Check sheet for the drawn part. Datum: minimum x, y, z corner. Units: mm. Give positions to 0.01 mm unless a question says otherwise; leave off trailing zeros. Loops run counter-clockwise (first coordinate to the right, second up) from the corner with the lowest first, then second, coordinate; pieces in that order, holes last.
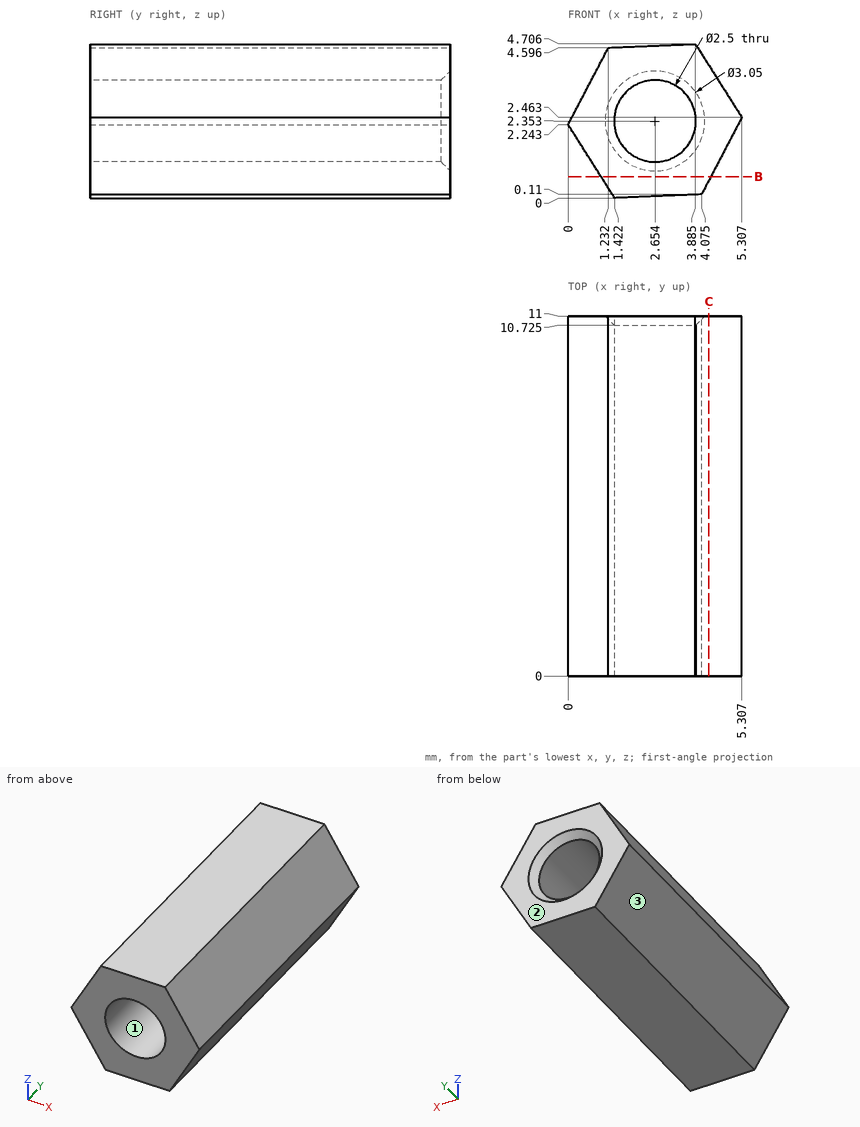
(1) Release check for a two-part mould opening along Z. For the marked faces 1, 2 and 3 record: pulls with the +Z half, pulls with the -Z half, needs draft (parallel to the pull), parting line crosses it, or undercut.
(2) Section check C-C on x = 4.3. Record the boundary of the cut face in (y, z).
(3) Material ranges on line 1 (Z direction, x = 1.7, y = 10) (1 decimal); line 2 (Z direction, x = 2.6, y = 9.25) (1 decimal); line 3 (X direction, y = 1.25, z = 3.35) (1 decimal), recorded low to high.
(4) Gauge pin test, flat end, axial feed: pin 1 Ø1 at (y, z) = (7, 1.5) entering from +X (1 decimal). Record the tip position at first contact, or that the pin passes through.
(5) Section check B-B on z = 0.65. Record the boundary of the cut face in (x, y).
Computed values:
1. face 1: undercut
1. face 2: needs draft
1. face 3: pulls with the -Z half
2. outline: (0, 0.54) - (11, 0.54) - (11, 4.05) - (0, 4.05) - close
3. line 1: z = 0 to 1.5, 3.2 to 4.6
3. line 2: z = 0 to 1.1, 3.6 to 4.7
3. line 3: x = 0.6 to 1.9, 3.4 to 4.7
4. pin 1: stops at x = 5.1
5. outline: (1.01, 0) - (4.36, 0) - (4.36, 11) - (1.01, 11) - close
